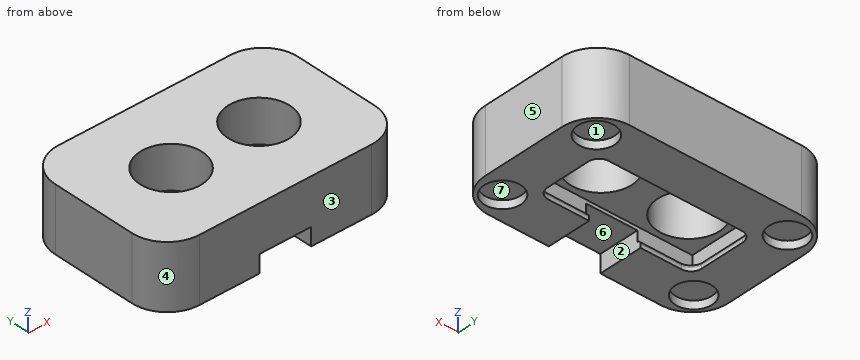
from build123d import *

# Parameters (mm, degrees)
SKETCH1_W           = 68.6
SKETCH1_H           = 43.8
SKETCH1_R           = 8.75
BOSS_EXTRUDE1_DEPTH = 12
CUT_EXTRUDE1_DEPTH  = 3.35
SKETCH3_W           = 68.6
SKETCH3_H           = 43.8
SKETCH3_W_2         = 45.6
SKETCH3_H_2         = 20.8
BOSS_EXTRUDE2_DEPTH = 6
FILLET1_R           = 10
SKETCH4_R           = 5.2
CUT_EXTRUDE2_DEPTH  = 2.3
BOSS_EXTRUDE6_DEPTH = 2
FILLET2_R           = 3
FILLET3_R           = 1
SKETCH7_W           = 14.55
SKETCH7_H           = 11.5
CUT_EXTRUDE3_DEPTH  = 5


with BuildPart() as part:
    # Sketch1 → Boss-Extrude1 (new body)
    with BuildSketch(Plane.XY):
        Rectangle(SKETCH1_W, SKETCH1_H)
        with Locations((12.415962636, 0)):
            Circle(SKETCH1_R, mode=Mode.SUBTRACT)
        with Locations(Location((-12.415962636, 0, 0), (0, 0, 180))):
            Circle(SKETCH1_R, mode=Mode.SUBTRACT)
    extrude(amount=BOSS_EXTRUDE1_DEPTH)

    # Sketch2 → Cut-Extrude1 (cut)
    with BuildSketch(Plane(origin=(0, 0, 0), x_dir=(-1, 0, 0), z_dir=(0, 0, -1))):
        with BuildLine():
            Line((3.175, 6), (-3.175, 6))
            ThreePointArc((-3.175, 6), (-5.3, 8.125), (-3.175, 10.25))
            Line((-3.175, 10.25), (3.175, 10.25))
            ThreePointArc((3.175, 10.25), (5.3, 8.125), (3.175, 6))
        make_face()
    extrude(amount=-CUT_EXTRUDE1_DEPTH, mode=Mode.SUBTRACT)

    # Sketch3 → Boss-Extrude2 (add)
    with BuildSketch(Plane(origin=(0, 0, 0), x_dir=(-1, 0, 0), z_dir=(0, 0, -1))):
        Rectangle(SKETCH3_W, SKETCH3_H)
        Rectangle(SKETCH3_W_2, SKETCH3_H_2, mode=Mode.SUBTRACT)
    extrude(amount=BOSS_EXTRUDE2_DEPTH)

    # Fillet1
    fillet1_edges = [part.edges().sort_by_distance(p)[0] for p in [
        (34.3, -21.9, 3),
        (-34.3, -21.9, 3),
        (-34.3, 21.9, 3),
        (34.3, 21.9, 3),
    ]]
    fillet(fillet1_edges, radius=FILLET1_R)

    # Sketch4 → Cut-Extrude2 (cut)
    with BuildSketch(Plane(origin=(0, 0, -6), x_dir=(-1, 0, 0), z_dir=(0, 0, -1))):
        with Locations((27, 14.6)):
            Circle(SKETCH4_R)
        with Locations(Location((-27, 14.6, 0), (0, 0, 180))):
            Circle(SKETCH4_R)
        with Locations(Location((27, -14.6, 0), (0, 0, 180))):
            Circle(SKETCH4_R)
        with Locations((-27, -14.6)):
            Circle(SKETCH4_R)
    extrude(amount=-CUT_EXTRUDE2_DEPTH, mode=Mode.SUBTRACT)

    # Sketch6 → Boss-Extrude6 (add)
    with BuildSketch(Plane(origin=(0, 0, -6), x_dir=(-1, 0, 0), z_dir=(0, 0, -1))):
        Polygon((-22.8, -10.4), (-7.275, -10.4), (-7.275, -9.4), (-21.8, -9.4), (-21.8, 9.4), (21.8, 9.4), (21.8, -9.4), (7.275, -9.4), (7.275, -10.4), (22.8, -10.4), (22.8, 10.4), (-22.8, 10.4), align=None)
    extrude(amount=-BOSS_EXTRUDE6_DEPTH)

    # Fillet2
    fillet2_edges = [part.edges().sort_by_distance(p)[0] for p in [
        (-21.8, -9.4, -5),
        (-21.8, 9.4, -5),
        (21.8, 9.4, -5),
        (21.8, -9.4, -5),
    ]]
    fillet(fillet2_edges, radius=FILLET2_R)

    # Fillet3
    fillet3_edges = [part.edges().sort_by_distance(p)[0] for p in [
        (13.0375, -9.4, -4),
        (20.921320344, -8.521320344, -4),
        (21.8, 0, -4),
        (20.921320344, 8.521320344, -4),
        (0, 9.4, -4),
        (-20.921320344, 8.521320344, -4),
        (-13.0375, -9.4, -4),
        (-20.921320344, -8.521320344, -4),
        (-21.8, 0, -4),
    ]]
    fillet(fillet3_edges, radius=FILLET3_R - 0.0001)  # a hair under: the kernel refuses the full size

    # Sketch7 → Cut-Extrude3 (cut)
    with BuildSketch(Plane(origin=(0, 0, -6), x_dir=(-1, 0, 0), z_dir=(0, 0, -1))):
        with Locations((0, -16.15)):
            Rectangle(SKETCH7_W, SKETCH7_H)
    extrude(amount=-CUT_EXTRUDE3_DEPTH, mode=Mode.SUBTRACT)


solid = part.part
The model under review builds one solid part; all positions refer to its coordinate system, in mm. Face numbers are marked on the shaded views. A direction names the side the tool comes from. Coordinates: 2 decimals unless noted, no trailing zeros. Loops run counter-clockwise (first coordinate to the right, second up) from the corner with the lowest first, then second, coordinate; pieces in that order, holes last. Notation, with made-up numbers: M 63,-26 L 67,-26 A26 cw 67,-9 Z; hole C 87,46.25 d4. An arc over 180 degrees is marked long. Put each result on its own line as item: value. Start each with the question number.
Q1. Wall thickness on line 1 (X direction, y = 11, z = -4.75); line 2 (Y direction, x = 19.5, z = -3.25); line 3 (X direction, y = 2, z = 8.5): over which ranges is each line inside the solid? List them lowest first.
Q2. Add section A-A (y = 0). Count the separate pieces of the cut face and the enclosed holes in it, and give its area (3 significant figures).
Q3. Add section B-B (z = 8). Write out the cut boundary in (x, y).
Q4. Add section D-D (z = -1.75). Write out the cut boundary in (x, y) (3 decimals), and give its area (3 significant figures).
Q5. Clearance check with flat-ended pins moving along their axes: pin 1 (3 mm diameter, centred on x = 29.5, y = -14.5, fed in from -Z); pin 2 (9 mm diameter, centred on x = -0.5, y = -13.5, fed in from -Z); pin 3 (1.5 mm diameter, centred on y = 13, z = -1.5, fed in from +X). State where each tip first meets the part, or that it passes through.
Q6. The part is to be moulded in two halves that separate along X. For the marked faces 1, 2, 3 and 4, say which applies: +X half, -X half, draft (parallel to the pull), parting line (faces both ways), or undercut.
Q7. For the marked faces 5, 6 and 7, list the 3-axis set-ups (+Z, -Z, +X, -X, +Y, -Y) from which the entire face can be reached by the end or side of a thin tool; tool diameter is ignored.
Answers:
1. line 1: x = -34.3 to -30.75, -23.25 to 23.25, 30.75 to 34.3
1. line 2: y = -21.9 to -10.4, 10.4 to 21.9
1. line 3: x = -34.3 to -20.93, -3.9 to 3.9, 20.93 to 34.3
2. separate pieces: 3
2. enclosed holes: 0
2. area: 545 mm^2
3. outline: M -34.3,-11.9 A10 ccw -24.3,-21.9 L 24.3,-21.9 A10 ccw 34.3,-11.9 L 34.3,11.9 A10 ccw 24.3,21.9 L -24.3,21.9 A10 ccw -34.3,11.9 Z; hole C -12.42,0 d17.5; hole C 12.42,0 d17.5
4. outline: M -34.3,-11.9 A10 ccw -24.3,-21.9 L -7.275,-21.9 L -7.275,-10.4 L -22.8,-10.4 L -22.8,10.4 L 22.8,10.4 L 22.8,-10.4 L 7.275,-10.4 L 7.275,-21.9 L 24.3,-21.9 A10 ccw 34.3,-11.9 L 34.3,11.9 A10 ccw 24.3,21.9 L -24.3,21.9 A10 ccw -34.3,11.9 Z
4. area: 1,800 mm^2
5. pin 1: stops at z = -3.7
5. pin 2: stops at z = -1
5. pin 3: stops at x = 34.29
6. face 1: undercut
6. face 2: undercut
6. face 3: draft
6. face 4: -X half
7. face 5: +Z, -Z, +X, +Y, -Y
7. face 6: -Z, -Y
7. face 7: -Z
